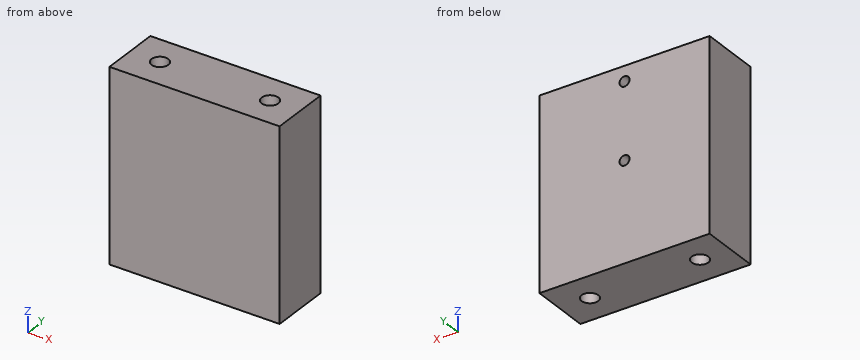
from build123d import *

# Parameters (mm, degrees)
SKIZZE1_W                       = 42.5
SKIZZE1_H                       = 15
AUFSATZ_LINEAR_AUSTRAGEN1_DEPTH = 47.5
M5_GEWINDEBOHRUNG1_D            = 4.2
M5_GEWINDEBOHRUNG1_DEPTH        = 10
M5_GEWINDEBOHRUNG1_TIP          = 1.2618073
M5_GEWINDEBOHRUNG2_D            = 4.2
M5_GEWINDEBOHRUNG2_DEPTH        = 10
M5_GEWINDEBOHRUNG2_TIP          = 1.2618073
M3_GEWINDEBOHRUNG1_D            = 2.5
M3_GEWINDEBOHRUNG1_DEPTH        = 8.5
M3_GEWINDEBOHRUNG1_TIP          = 0.751075774


with BuildPart() as part:
    # Skizze1 → Aufsatz-Linear austragen1 (new body)
    with BuildSketch(Plane.XY):
        with Locations((21.25, 7.5)):
            Rectangle(SKIZZE1_W, SKIZZE1_H)
    extrude(amount=AUFSATZ_LINEAR_AUSTRAGEN1_DEPTH)

    # M5 Gewindebohrung1
    with Locations(Plane(origin=(0, 0, 0), x_dir=(-1, 0, 0), z_dir=(0, 0, -1))):
        with Locations((-7.5, 7.5), (-35, 7.5)):
            Hole(M5_GEWINDEBOHRUNG1_D / 2, depth=M5_GEWINDEBOHRUNG1_DEPTH)
            with Locations((0, 0, -(M5_GEWINDEBOHRUNG1_DEPTH + M5_GEWINDEBOHRUNG1_TIP / 2))):  # 118° drill point
                Cone(0, M5_GEWINDEBOHRUNG1_D / 2, M5_GEWINDEBOHRUNG1_TIP, mode=Mode.SUBTRACT)

    # M5 Gewindebohrung2
    with Locations(Plane(origin=(7.5, 7.5, 47.5), x_dir=(1, 0, 0), z_dir=(0, 0, 1))):
        with Locations((0, 0), (27.5, 0)):
            Hole(M5_GEWINDEBOHRUNG2_D / 2, depth=M5_GEWINDEBOHRUNG2_DEPTH)
            with Locations((0, 0, -(M5_GEWINDEBOHRUNG2_DEPTH + M5_GEWINDEBOHRUNG2_TIP / 2))):  # 118° drill point
                Cone(0, M5_GEWINDEBOHRUNG2_D / 2, M5_GEWINDEBOHRUNG2_TIP, mode=Mode.SUBTRACT)

    # M3 Gewindebohrung1
    with Locations(Plane(origin=(21.25, 15, 43.75), x_dir=(0, 0, 1), z_dir=(0, 1, 0))):
        with Locations((0, 0), (-19, 0)):
            Hole(M3_GEWINDEBOHRUNG1_D / 2, depth=M3_GEWINDEBOHRUNG1_DEPTH)
            with Locations((0, 0, -(M3_GEWINDEBOHRUNG1_DEPTH + M3_GEWINDEBOHRUNG1_TIP / 2))):  # 118° drill point
                Cone(0, M3_GEWINDEBOHRUNG1_D / 2, M3_GEWINDEBOHRUNG1_TIP, mode=Mode.SUBTRACT)


solid = part.part
Read the model definition and answer for the solid it produces. Units are mm, in the model's axes. Give positions to 0.01 mm unless a question says otherwise; leave off trailing zeros. Loops run counter-clockwise (first coordinate to the right, second up) from the corner with the lowest first, then second, coordinate; pieces in that order, holes last. Notation, with made-up numbers: M 8.5,89.25 L 41.5,89.25 A19 cw 41.5,99.25 Z; hole C 50,-12.5 d9. An arc over 180 degrees is marked long. Write each question's results on one line, items separated by ' | '.
1. Straight lines are drawn through the part: line 1 (Z direction, x = 21.25, y = 11.5); line 2 (X direction, y = 7.5, z = 40.5); line 3 (X direction, y = 10.25, z = 24.75). For each, find the intervals that lie inside material, in ascending order. Write a range as [from, to].
Values:
line 1: z = [0, 23.5], [26, 42.5], [45, 47.5] | line 2: x = [0, 5.4], [9.6, 32.9], [37.1, 42.5] | line 3: x = [0, 20], [22.5, 42.5]
2. Section A-A on z = 6.5 is taken. Give the vertices of the cut face in (x, y), plus the area to 3 significant figures.
Values:
outline: M 0,0 L 42.5,0 L 42.5,15 L 0,15 Z; hole C 7.5,7.5 d4.2; hole C 35,7.5 d4.2 | area: 610 mm^2
3. Section B-B on y = 8.5 is taken. State how many separate pieces and enclosed holes the cut face has, plus the area to 3 significant figures.
Values:
separate pieces: 1 | enclosed holes: 2 | area: 1,860 mm^2
